Here's how the part is built. I have some questions about the finished solid (model axes, mm). Coordinates: 2 decimals unless noted, no trailing zeros. Loops run counter-clockwise (first coordinate to the right, second up) from the corner with the lowest first, then second, coordinate; pieces in that order, holes last. Notation, with made-up numbers: M -4.75,-35.75 L 7.25,-35.75 A10 cw 7.25,-22.75 Z; hole C 44.5,22 d2. An arc over 180 degrees is marked long. Use one line per item in the form item = value. Start each with the question number.
(1) Imagine slicing it at A-A, the plane z = -17.5. Please give me the cut outline in (x, y), and give its area (3 significant figures).
(2) Please list where these lines run through material, in increasing order: L1, parallel to X at y = 2.05, z = 17.5; L2, parallel to Z at x = 12, y = 0.8; L3, parallel to X at y = 2.05, z = 0.
(3) Imagine slicing it at B-B, the plane y = 2.2. Please give me the cut outline in (x, z), and give its area (3 significant figures).
(4) Imagine slicing it at C-C, the plane x = -12. Please give me the cut outline in (y, z).
(5) Imagine slicing it at D-D, the plane x = 1. Please give me the cut outline in (y, z), and give its area (3 significant figures).
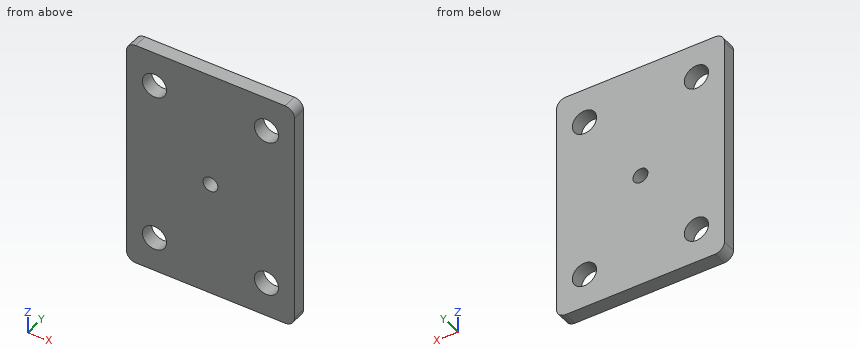
```python
from build123d import *

# Parameters (mm, degrees)
SKETCH_1_W          = 36
SKETCH_1_H          = 50
SKETCH_1_R          = 2.6
EXTRUDE_1_DEPTH     = 3
FILLET_1_R          = 2
SKETCH_6_R          = 1.6
CUT_EXTRUDE_5_DEPTH = 10


with BuildPart() as part:
    # 草图1 → 凸台-拉伸1 (new body)
    with BuildSketch(Plane(origin=(0, 0, 0), x_dir=(1, 0, 0), z_dir=(0, 1, 0))):
        Rectangle(SKETCH_1_W, SKETCH_1_H)
        with Locations((-12, 17.5)):
            Circle(SKETCH_1_R, mode=Mode.SUBTRACT)
        with Locations((12, 17.5)):
            Circle(SKETCH_1_R, mode=Mode.SUBTRACT)
        with Locations((-12, -17.5)):
            Circle(SKETCH_1_R, mode=Mode.SUBTRACT)
        with Locations((12, -17.5)):
            Circle(SKETCH_1_R, mode=Mode.SUBTRACT)
    extrude(amount=EXTRUDE_1_DEPTH)

    # 圆角1
    fillet_1_edges = [part.edges().sort_by_distance(p)[0] for p in [
        (18, 1.5, 25),
        (-18, 1.5, 25),
        (-18, 1.5, -25),
        (18, 1.5, -25),
    ]]
    fillet(fillet_1_edges, radius=FILLET_1_R)

    # 草图6 → 切除-拉伸5 (cut)
    with BuildSketch(Plane(origin=(0, 3, 0), x_dir=(1, 0, 0), z_dir=(0, 1, 0))):
        Circle(SKETCH_6_R)
    extrude(amount=-CUT_EXTRUDE_5_DEPTH, mode=Mode.SUBTRACT)


solid = part.part
```
Answer:
q1.outline = M -18,0 L -14.6,0 L -14.6,3 L -18,3 Z; M -9.4,0 L 9.4,0 L 9.4,3 L -9.4,3 Z; M 14.6,0 L 18,0 L 18,3 L 14.6,3 Z
q1.area = 76.8 mm²
q2.L1 = -18 to -14.6, -9.4 to 9.4, 14.6 to 18
q2.L2 = -25 to -20.1, -14.9 to 14.9, 20.1 to 25
q2.L3 = -18 to -1.6, 1.6 to 18
q3.outline = M -18,-23 A2 ccw -16,-25 L 16,-25 A2 ccw 18,-23 L 18,23 A2 ccw 16,25 L -16,25 A2 ccw -18,23 Z; hole C -12,-17.5 d5.2; hole C -12,17.5 d5.2; hole C 0,0 d3.2; hole C 12,-17.5 d5.2; hole C 12,17.5 d5.2
q3.area = 1,700 mm²
q4.outline = M 0,-25 L 3,-25 L 3,-20.1 L 0,-20.1 Z; M 0,-14.9 L 3,-14.9 L 3,14.9 L 0,14.9 Z; M 0,20.1 L 3,20.1 L 3,25 L 0,25 Z
q5.outline = M 0,-25 L 3,-25 L 3,-1.25 L 0,-1.25 Z; M 0,1.25 L 3,1.25 L 3,25 L 0,25 Z
q5.area = 143 mm²
